The model under review builds one solid part; all positions refer to its coordinate system, in mm. A direction names the side the tool comes from. Coordinates: 2 decimals unless noted, no trailing zeros. Loops run counter-clockwise (first coordinate to the right, second up) from the corner with the lowest first, then second, coordinate; pieces in that order, holes last. Notation, with made-up numbers: M 44,-12.75 L 87,-12.75 A14 cw 87,12.25 Z; hole C 55.5,-23.5 d7. An arc over 180 degrees is marked long. Return JSON: item names as keys, results as strings.
```python
from build123d import *

# Parameters (mm, degrees)
BOSS_EXTRUDE2_DEPTH = 2.5
CUT_EXTRUDE5_DEPTH  = 3.5
CUT_EXTRUDE7_DEPTH  = 3.5
SKETCH8_R           = 1.6
CUT_EXTRUDE8_DEPTH  = 3.5


with BuildPart() as part:
    # Sketch1 → Boss-Extrude2 (new body)
    with BuildSketch(Plane(origin=(0, 0, 0), x_dir=(1, 0, 0), z_dir=(0, 1, 0))):
        with BuildLine():
            Line((0, 0), (-70, 0))
            Line((-70, 0), (-70, 290))
            Line((-70, 290), (0, 290))
            ThreePointArc((0, 290), (102.530483272, 247.530483272), (145, 145))
            Line((145, 145), (145, 0))
            Line((145, 0), (0, 0))
        make_face()
    extrude(amount=BOSS_EXTRUDE2_DEPTH)

    # Sketch6 → Cut-Extrude5 (cut, through all)
    with BuildSketch(Plane(origin=(0, 0, 0), x_dir=(1, 0, 0), z_dir=(0, 1, 0))):
        Polygon((5.773502692, 135), (11.547005384, 145), (5.773502692, 155), (-5.773502692, 155), (-11.547005384, 145), (-5.773502692, 135), align=None)
    extrude(amount=CUT_EXTRUDE5_DEPTH, mode=Mode.SUBTRACT)

    # Sketch7 → Cut-Extrude7 (cut, through all)
    with BuildSketch(Plane(origin=(0, 0, 0), x_dir=(1, 0, 0), z_dir=(0, 1, 0))):
        with BuildLine():
            ThreePointArc((-32.352380638, 24.259271714), (0, 20), (32.352380638, 24.259271714))
            ThreePointArc((32.352380638, 24.259271714), (50.030050167, 54.877893499), (19.411428383, 72.555563028))
            ThreePointArc((19.411428383, 72.555563028), (0, 70), (-19.411428383, 72.555563028))
            ThreePointArc((-19.411428383, 72.555563028), (-50.030050167, 54.877893499), (-32.352380638, 24.259271714))
        make_face()
    extrude(amount=CUT_EXTRUDE7_DEPTH, mode=Mode.SUBTRACT)

    # Sketch8 → Cut-Extrude8 (cut, through all)
    with BuildSketch(Plane(origin=(0, 0, 0), x_dir=(1, 0, 0), z_dir=(0, 1, 0))):
        with Locations((-20, 15)):
            Circle(SKETCH8_R)
        with Locations((20, 15)):
            Circle(SKETCH8_R)
    extrude(amount=CUT_EXTRUDE8_DEPTH, mode=Mode.SUBTRACT)


solid = part.part
```
1. Add section B-B on z = -59.5. Give the boundary of the cut face in (x, y), plus the area to 3 significant figures.
Check values:
{"outline": "M -70,0 L -48.29,0 L -48.29,2.5 L -70,2.5 Z; M 48.29,0 L 145,0 L 145,2.5 L 48.29,2.5 Z", "area": "296 mm²"}
2. Add section D-D on z = -205.5. Give the boundary of the cut face in (x, y).
Check values:
{"outline": "M -70,0 L 131.78,0 L 131.78,2.5 L -70,2.5 Z"}
3. To check wall thickness, follow line 1 (Z direction, x = -1, y = 0.2); line 2 (X direction, y = 0.7, z = -15); line 3 (Z direction, x = 20, y = 0.65). State the ranges of each line that lie inside material, in increasing order.
Check values:
{"line 1": "-290 to -155, -135 to -70.01, -20 to 0", "line 2": "-70 to -21.6, -18.4 to 18.4, 21.6 to 145", "line 3": "-288.61 to -72.71, -21.61 to -16.6, -13.4 to 0"}
4. The part is to be moulded in two halves that separate along Z. For faces 3 (the face through (39, 2.5, -147)), 4 (the face through (101.4, 1.23, -248.65)), 5 (the face through (8.7, 1.23, -149.93)), say which applies: released by +Z, released by -Z, zero draft, split by the parting line, or undercut.
Check values:
{"face 3": "zero draft", "face 4": "released by -Z", "face 5": "undercut"}
5. Insertion check: pin 1 Ø4 at (x, z) = (20, -15) entering from -Y; pin 2 Ø1.5 at (y, z) = (0.5, -231) entering from +X. Each pin has a flat end and moves straight along its axis. Give the tip position at first contact, or say it passes through.
Check values:
{"pin 1": "y = 0", "pin 2": "x = 117.29"}
6. Add section A-A on y = 1.65. Give the boundary of the cut face in (x, z).
Check values:
{"outline": "M -70,-290 L 0,-290 A145 ccw 145,-145 L 145,0 L -70,0 Z; hole M -32.35,-24.26 A25 ccw -19.41,-72.56 A75 cw 19.41,-72.56 A25 ccw 32.35,-24.26 A125 ccw Z; hole C -20,-15 d3.2; hole M -11.55,-145 L -5.77,-155 L 5.77,-155 L 11.55,-145 L 5.77,-135 L -5.77,-135 Z; hole C 20,-15 d3.2"}
7. Add section C-C on x = 44. Give the boundary of the cut face in (y, z), plus the area to 3 significant figures.
Check values:
{"outline": "M 0,-283.16 L 2.5,-283.16 L 2.5,-65.63 L 0,-65.63 Z; M 0,-31.18 L 2.5,-31.18 L 2.5,0 L 0,0 Z", "area": "622 mm²"}
8. Machinability: for faces 1 (the face through (39, 0, -147)), 2 (the face through (-8.7, 1.23, -140.07)), which of the approach directions +Z, -Z, +X, -X, +Y, -Y give a long, thin tool a straight path to every point of the face, cutting with its end or side? Answer none if there is none.
Check values:
{"face 1": "+Z, -Z, +X, -X, -Y", "face 2": "+Y, -Y"}
